Geometry: final body of the model. Coordinates: model frame, mm. Face numbers are marked on the shaded views. A direction names the side the tool comes from. Coordinates: 2 decimals unless noted, no trailing zeros. Order: outer loops, then holes, each group sorted by start corner. A loop starts at its lowest first (then second) coordinate and runs counter-clockwise, first axis right, second up. Notation, with made-up numbers: M 16.25,13.5 L 34.25,13.5 A22 ccw 34.25,50.5 Z; hole C 10,30.5 d6. An arc over 180 degrees is marked long. One line per question, with ' | ' between items.
Autodesk Inventor part; units mm, degrees
ref_plane "YZ Plane" through (0, 0, 0) normal (1, 0, 0) x (0, 1, 0)
ref_plane "XZ Plane" through (0, 0, 0) normal (0, 1, 0) x (-1, 0, 0)
ref_plane "XY Plane" through (0, 0, 0) normal (0, 0, 1) x (1, 0, 0)
sketch "Skizze1" plane through (0, 0, 0) normal (0, 0, 1) x (1, 0, 0)
  line L0 (-34.16, 0) -> (34.16, 0) construction
  circle A0 centre (0, 0) radius 19.4 construction
  circle A1 centre (0, 19.4) radius 1.15
  circle A2 centre (16.8009, -9.7) radius 1.15
  circle A3 centre (-16.8009, -9.7) radius 1.15
  line L1 (0, 34.16) -> (0, -34.16) construction
  line L2 (0, 0) -> (-16.8009, -9.7) construction
  circle A4 centre (0, 0) radius 14.4
  circle A5 centre (0, 0) radius 24.4
  circle A6 centre (16.8009, -9.7) radius 2.85
  circle A7 centre (0, 19.4) radius 2.85
  circle A8 centre (-16.8009, -9.7) radius 2.85
  circle A9 centre (0, 19.4) radius 4.5
  circle A10 centre (16.8009, -9.7) radius 4.5
  circle A11 centre (-16.8009, -9.7) radius 4.5
  dimension "d0" = 38.8
  dimension "d1" = 2.3
  dimension "d2" = 30
  dimension "d3" = 5
  dimension "d4" = 5
  dimension "d21" = 5.7
  dimension "d27" = 9
extrude "Extrusion2" add sketch "Skizze1" along normal blind 3 contours A5 | A6 | A7 | A8 | A9 | A10 | A11
extrude "Extrusion4" add sketch "Skizze1" along normal blind 3 from surface at 3 contours A6 | A7 | A8 | A9 | A10 | A11
extrude "Extrusion5" add sketch "Skizze1" along normal blind 3 from surface at 6 contours A6 | A7 | A8
extrude "Extrusion6" cut sketch "Skizze1" along normal blind 2 contours A6 | A7 | A8
equation "\"d3\" = d4"
properties part number "PlanetaryHolderBottom"
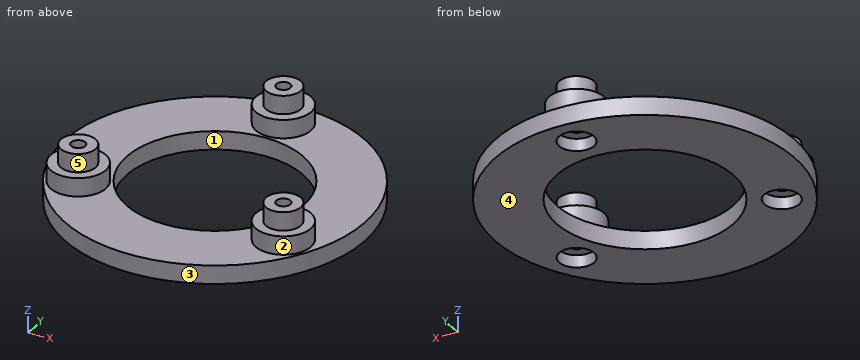
1. Section C-C, the plane y = 0. Output: boundary loops of the cut face in (x, z), and give its area (3 significant figures).
Response values:
outline: M -24.4,0 L -14.4,0 L -14.4,3 L -24.4,3 Z; M 14.4,0 L 24.4,0 L 24.4,3 L 14.4,3 Z | area: 60.0 mm^2
2. Section A-A, the plane z = 4.5. Output: boundary loops of the cut face in (x, y).
Response values:
outline: C -16.8,-9.7 d9; C 0,19.4 d9; C 16.8,-9.7 d9; hole C -16.8,-9.7 d2.3; hole C 0,19.4 d2.3; hole C 16.8,-9.7 d2.3
3. Section B-B, the plane x = 0. Output: boundary loops of the cut face in (y, z), and give its area (3 significant figures).
Response values:
outline: M -24.4,0 L -14.4,0 L -14.4,3 L -24.4,3 Z; M 14.4,0 L 16.55,0 L 16.55,2 L 18.25,2 L 18.25,9 L 16.55,9 L 16.55,6 L 14.9,6 L 14.9,3 L 14.4,3 Z; M 20.55,2 L 22.25,2 L 22.25,0 L 24.4,0 L 24.4,3 L 23.9,3 L 23.9,6 L 22.25,6 L 22.25,9 L 20.55,9 Z | area: 76.6 mm^2
4. Section D-D, the plane x = -5.5. Output: boundary loops of the cut face in (y, z), and give its area (3 significant figures).
Response values:
outline: M -23.77,0 L -13.31,0 L -13.31,3 L -23.77,3 Z; M 13.31,0 L 23.77,0 L 23.77,3 L 13.31,3 Z | area: 62.8 mm^2
5. Draft query along X for the marked faces 3, 4 and 5. Return one class per face: pulls with the +X half, pulls with the -X half, needs draft (parallel to the pull), parting line crosses it, or undercut.
Response values:
face 3: parting line crosses it | face 4: needs draft | face 5: undercut
6. Material intervals for line 1 (Y direction, x = -0.5, z = 2.5); line 2 (Y direction, x = 0, z = 4.75); line 3 (Z direction, x = -12, y = 16), sorted ascending. Write a range as [from, to].
Response values:
line 1: y = [-24.39, -14.39], [14.39, 18.36], [20.44, 24.39] | line 2: y = [14.9, 18.25], [20.55, 23.9] | line 3: z = [0, 3]
7. Access query for the marked faces 1 and 2. Directions: +Z, -Z, +X, -X, +Y, -Y. A direction counts if a zero-diameter tool reaches every point of the face in a straight line with its end or side. Return the directions, or none.
Response values:
face 1: +Z, -Z | face 2: +Z
8. Pin query (flat end, axial travel): P1, Ø1.7, axis at x = -0.5, y = 18.5, coming from the -Z side; P2, Ø7.5, axis at x = 16.8, y = -9.7, coming from the +Z side; P3, Ø1.5, axis at x = 1.5, y = -14, coming from the +Z side; P4, Ø1.8, axis at x = -16.8, y = -9.7, coming from the -Z side. Return the tip coordinate at first contact, or that it passes through.
Response values:
P1: stops at z = 2 | P2: stops at z = 9 | P3: stops at z = 3 | P4: passes through
